```python
from build123d import *
from OCP.BRepFilletAPI import BRepFilletAPI_MakeChamfer

# Parameters (mm, degrees)
MAIN_BODY_DEPTH            = 15
F_12_0_12_DIAMETER_HOLE1_D = 12
M12X1_75_TAPPED_HOLE2_D    = 10.2
SKETCH4_W                  = 30
SKETCH4_H                  = 13
CUT_OUT_DEPTH              = 139.740765458
C_FER_5_X_45_SIZE          = 5
C_FER_3_X_30_SIZE          = 3
C_FER_3_X_30_SIZE2         = 5.196152423


with BuildPart() as part:
    # Sketch1 → main body (new, symmetric)
    with BuildSketch(Plane.XY):
        with BuildLine():
            Line((20, 0), (-130, 0))
            Line((-130, 0), (-130, 40))
            Line((-130, 40), (132, 40))
            Line((132, 40), (132, 20))
            Line((132, 20), (76.568542495, 20))
            ThreePointArc((76.568542495, 20), (46.568542495, 14.852813742), (20, 0))
        make_face()
    extrude(amount=MAIN_BODY_DEPTH, both=True)

    # Ø12.0 (12) Diameter Hole1 (through all)
    with Locations(Plane(origin=(-115, 20, 15), x_dir=(1, 0, 0), z_dir=(0, 0, 1))):
        with Locations((0, 0)):
            Hole(F_12_0_12_DIAMETER_HOLE1_D / 2)

    # M12x1.75 Tapped Hole2 (through all)
    with Locations(Plane(origin=(0, 40, 0), x_dir=(-1, 0, 0), z_dir=(0, 1, 0))):
        with Locations((0, 0)):
            Hole(M12X1_75_TAPPED_HOLE2_D / 2)

    # Sketch4 → cut out (cut, through all)
    with BuildSketch(Plane(origin=(0, 40, 0), x_dir=(1, 0, 0), z_dir=(0, 1, 0))):
        with Locations((117, 0)):
            Rectangle(SKETCH4_W, SKETCH4_H)
    extrude(amount=-CUT_OUT_DEPTH, mode=Mode.SUBTRACT)

    # C'FER 5 x 45
    c_fer_5_x_45_edges = [part.edges().sort_by_distance(p)[0] for p in [
        (-130, 40, 0),
    ]]
    chamfer(c_fer_5_x_45_edges, length=C_FER_5_X_45_SIZE)

    # C'FER 3 x 30: one chamfer whose edges measure the first distance from different faces: ONE call of the kernel's chamfer builder (chamfer() names one face for all edges)
    c_fer_3_x_30_edges_1 = [part.edges().sort_by_distance(p)[0] for p in [
        (132, 30, -6.5),
    ]]
    c_fer_3_x_30_side_1 = [part.faces().sort_by_distance(p)[0] for p in [
        (132, 30, -10.75),
    ]]
    c_fer_3_x_30_edges_2 = [part.edges().sort_by_distance(p)[0] for p in [
        (132, 30, 6.5),
    ]]
    c_fer_3_x_30_side_2 = [part.faces().sort_by_distance(p)[0] for p in [
        (132, 30, 10.75),
    ]]
    c_fer_3_x_30 = BRepFilletAPI_MakeChamfer(part.part.solid().wrapped)
    for e in c_fer_3_x_30_edges_1:
        c_fer_3_x_30.Add(C_FER_3_X_30_SIZE, C_FER_3_X_30_SIZE2, e.wrapped, c_fer_3_x_30_side_1[0].wrapped)  # the first distance lies on this face
    for e in c_fer_3_x_30_edges_2:
        c_fer_3_x_30.Add(C_FER_3_X_30_SIZE, C_FER_3_X_30_SIZE2, e.wrapped, c_fer_3_x_30_side_2[0].wrapped)  # the first distance lies on this face
    add(Compound.cast(c_fer_3_x_30.Shape()), mode=Mode.REPLACE)


solid = part.part
```
Could you check a few things on this model? Use its own coordinates, in mm. A direction names the side the tool comes from. Give positions to 0.01 mm unless a question says otherwise; leave off trailing zeros. Loops run counter-clockwise (first coordinate to the right, second up) from the corner with the lowest first, then second, coordinate; pieces in that order, holes last. Notation, with made-up numbers: (-22.75, 11.5) - (33.25, 11.5) arc R34 cw to (33.25, 45.5) - close; hole circle Ø6 at (-8, -8.75). An arc over 180 degrees is marked (long way). Answer in a Markdown table with one row per item. Add a question column.
Q1. If we section it at A-A (z = 0): List the corners of the cut face in (x, y) for me.
Q2. We'd pull the mould along Z, two halves only. Please class faces 4 (the face through (129.4, 30.1, -8)), 5 (the face through (3, 25, -15)), 6 (the face through (-130, 17, 0)): +Z half, -Z half, draft (parallel to the pull), parting line (faces both ways), or undercut.
Q3. If we section it at B-B (x = -115): List the corners of the cut face in (y, z) for me, plus the area to 3 significant figures.
Q4. Please list where these lines run through material, in increasing order: L1, parallel to Z at x = 0, y = 15; L2, parallel to X at y = 22.5, z = -0.25; L3, parallel to Y at x = -115, z = 1. Write a range as from..to.
Q5. Which directions (+Z, -Z, +X, -X, +Y, -Y) give clear straight access to the entire face, cutting with the end or side of a thin tool? Please do faces 1 (the face through (114, 30, -6.5)), 2 (the face through (-127, 38, 0)), 3 (the face through (99, 20, 0)).
Q6. For pin 1 (15 mm diameter, centred on x = 112, z = -0.5, fed in from -Y); pin 2 (6 mm diameter, centred on y = 9, z = 6.5, fed in from +X); pin 3 (10.5 mm diameter, centred on y = 27, z = 0.5, fed in from +X); pin 4 (2 mm diameter, centred on x = 3, z = 1.5, fed in from +Y), each with a flat end and sliding along its axis, tell me the tip position at first contact or that it passes through.
Q7. If we section it at C-C (y = 11): List the corners of the cut face in (x, z) for me, plus the area to 3 significant figures.
Q8. If we section it at D-D (x = 0): List the corners of the cut face in (y, z) for me.
The answers:
| question | item | result |
|---|---|---|
| 1 | outline | (-130, 0) - (-5.1, 0) - (-5.1, 40) - (-125, 40) - (-130, 35) - close; (5.1, 0) - (20, 0) arc R90 cw to (76.57, 20) - (102, 20) - (102, 40) - (5.1, 40) - close; hole circle Ø12 at (-115, 20) |
| 2 | face 4 | undercut |
| 2 | face 5 | -Z half |
| 2 | face 6 | draft |
| 3 | outline | (0, -15) - (14, -15) - (14, 15) - (0, 15) - close; (26, -15) - (40, -15) - (40, 15) - (26, 15) - close |
| 3 | area | 840 mm^2 |
| 4 | L1 | z = -15..-5.1, 5.1..15 |
| 4 | L2 | x = -130..-120.45, -109.55..-5.09, 5.09..102 |
| 4 | L3 | y = 0..14, 26..40 |
| 5 | face 1 | +X, +Y, -Y |
| 5 | face 2 | +Z, -Z, -X, +Y |
| 5 | face 3 | +Z, -Z, +X, -Y |
| 6 | pin 1 | stops at y = 20 |
| 6 | pin 2 | stops at x = 39.47 |
| 6 | pin 3 | stops at x = 102 |
| 6 | pin 4 | passes through |
| 7 | outline | (-130, -15) - (37.34, -15) - (37.34, 15) - (-130, 15) - close; hole circle Ø10.2 at (0, 0) |
| 7 | area | 4,940 mm^2 |
| 8 | outline | (0, -15) - (40, -15) - (40, -5.1) - (0, -5.1) - close; (0, 5.1) - (40, 5.1) - (40, 15) - (0, 15) - close |
